from build123d import *

# Parameters (mm, degrees)
BOSS_EXTRUDE1_DEPTH = 77.15
CUT_EXTRUDE1_REACH  = 208.975
SKETCH2_R           = 1.75
SKETCH2_W           = 37
SKETCH2_H           = 18
FILLET1_R           = 2
FILLET2_R           = 10
SKETCH6_OUTSIDE_W   = 125.596
SKETCH6_OUTSIDE_H   = 125.596
SKETCH6_OUTSIDE_W_2 = 77.15
SKETCH6_OUTSIDE_H_2 = 77.15
SKETCH6_OUTSIDE_R   = 2.1
SKETCH6_OUTSIDE_R_2 = 2.55
CUT_EXTRUDE2_DEPTH  = 5


with BuildPart() as part:
    # Sketch1 → Boss-Extrude1 (new body)
    with BuildSketch(Plane.XY):
        Polygon((-29.117903226, 28.371290323), (-29.117903226, -48.778709677), (-24.117903226, -48.778709677), (-24.117903226, 23.371290323), (175.882096774, 23.371290323), (175.882096774, 28.371290323), align=None)
    extrude(amount=BOSS_EXTRUDE1_DEPTH)

    # Sketch2 → Cut-Extrude1 (cut, up to next)
    with BuildSketch(Plane(origin=(0, 28.371290323, 0), x_dir=(1, 0, 0), z_dir=(0, 1, 0)), mode=Mode.PRIVATE) as cut_extrude1_sk1:
        with Locations(Location((169.632096774, -38.575, 0), (0, 0, 180))):
            Circle(SKETCH2_R)
    cut_extrude1_tool1 = extrude(cut_extrude1_sk1.sketch, amount=-CUT_EXTRUDE1_REACH, mode=Mode.PRIVATE) & part.part
    # Sketch2 → Cut-Extrude1 (cut, up to next)
    with BuildSketch(Plane(origin=(0, 28.371290323, 0), x_dir=(1, 0, 0), z_dir=(0, 1, 0)), mode=Mode.PRIVATE) as cut_extrude1_sk2:
        with Locations(Location((117.632096774, -38.575, 0), (0, 0, 180))):
            Circle(SKETCH2_R)
    cut_extrude1_tool2 = extrude(cut_extrude1_sk2.sketch, amount=-CUT_EXTRUDE1_REACH, mode=Mode.PRIVATE) & part.part
    # Sketch2 → Cut-Extrude1 (cut, up to next)
    with BuildSketch(Plane(origin=(0, 28.371290323, 0), x_dir=(1, 0, 0), z_dir=(0, 1, 0)), mode=Mode.PRIVATE) as cut_extrude1_sk3:
        Polygon((175.882096774, -13.575), (115.882096774, -13.575), (-29.117903226, 0), (175.882096774, 0), align=None)
    cut_extrude1_tool3 = extrude(cut_extrude1_sk3.sketch, amount=-CUT_EXTRUDE1_REACH, mode=Mode.PRIVATE) & part.part
    # Sketch2 → Cut-Extrude1 (cut, up to next)
    with BuildSketch(Plane(origin=(0, 28.371290323, 0), x_dir=(1, 0, 0), z_dir=(0, 1, 0)), mode=Mode.PRIVATE) as cut_extrude1_sk4:
        Polygon((175.882096774, -63.575), (115.882096774, -63.575), (-29.117903226, -77.15), (175.882096774, -77.15), align=None)
    cut_extrude1_tool4 = extrude(cut_extrude1_sk4.sketch, amount=-CUT_EXTRUDE1_REACH, mode=Mode.PRIVATE) & part.part
    # Sketch2 → Cut-Extrude1 (cut, up to next)
    with BuildSketch(Plane(origin=(0, 28.371290323, 0), x_dir=(1, 0, 0), z_dir=(0, 1, 0)), mode=Mode.PRIVATE) as cut_extrude1_sk5:
        with Locations((146.882096774, -38.575)):
            Rectangle(SKETCH2_W, SKETCH2_H)
    cut_extrude1_tool5 = extrude(cut_extrude1_sk5.sketch, amount=-CUT_EXTRUDE1_REACH, mode=Mode.PRIVATE) & part.part
    add(cut_extrude1_tool1.solids().sort_by_distance((169.632097, 28.37129, 38.575))[0], mode=Mode.SUBTRACT)
    add(cut_extrude1_tool2.solids().sort_by_distance((117.632097, 28.37129, 38.575))[0], mode=Mode.SUBTRACT)
    add(cut_extrude1_tool3.solids().sort_by_distance((103.020462, 28.37129, 5.549528))[0], mode=Mode.SUBTRACT)
    add(cut_extrude1_tool4.solids().sort_by_distance((103.020462, 28.37129, 71.600472))[0], mode=Mode.SUBTRACT)
    add(cut_extrude1_tool5.solids().sort_by_distance((146.882097, 28.37129, 38.575))[0], mode=Mode.SUBTRACT)

    # Fillet1
    fillet1_edges = [part.edges().sort_by_distance(p)[0] for p in [
        (-29.117903226, 28.371290323, 38.575),
        (-24.117903226, 23.371290323, 38.575),
        (128.382096774, 25.871290323, 47.575),
        (128.382096774, 25.871290323, 29.575),
        (165.382096774, 25.871290323, 29.575),
        (165.382096774, 25.871290323, 47.575),
    ]]
    fillet(fillet1_edges, radius=FILLET1_R)

    # Fillet2
    fillet2_edges = [part.edges().sort_by_distance(p)[0] for p in [
        (175.882096774, 25.871290323, 13.575),
        (175.882096774, 25.871290323, 63.575),
    ]]
    fillet(fillet2_edges, radius=FILLET2_R)

    # Sketch6 outside → Cut-Extrude2 (cut)
    # profile 1 of 6: a face of its own
    with BuildSketch(Plane.ZY.offset(29.117903226)):
        with Locations((38.575, -10.204)):
            Rectangle(SKETCH6_OUTSIDE_W, SKETCH6_OUTSIDE_H)
        with Locations((38.575, -10.203709677)):
            Rectangle(SKETCH6_OUTSIDE_W_2, SKETCH6_OUTSIDE_H_2, mode=Mode.SUBTRACT)
    # profile 2 of 6: a face of its own
    with BuildSketch(Plane.ZY.offset(29.117903226)):
        with Locations((8.575, -20.203709677)):
            Circle(SKETCH6_OUTSIDE_R)
    # profile 3 of 6: a face of its own
    with BuildSketch(Plane.ZY.offset(29.117903226)):
        with Locations((8.575, -0.203709677)):
            Circle(SKETCH6_OUTSIDE_R)
    # profile 4 of 6: a face of its own
    with BuildSketch(Plane.ZY.offset(29.117903226)):
        with Locations((38.575, -40.203709677)):
            Circle(SKETCH6_OUTSIDE_R_2)
    # profile 5 of 6: a face of its own
    with BuildSketch(Plane.ZY.offset(29.117903226)):
        with Locations((68.575, -20.203709677)):
            Circle(SKETCH6_OUTSIDE_R)
    # profile 6 of 6: a face of its own
    with BuildSketch(Plane.ZY.offset(29.117903226)):
        with Locations((68.575, -0.203709677)):
            Circle(SKETCH6_OUTSIDE_R)
    extrude(amount=-CUT_EXTRUDE2_DEPTH, mode=Mode.SUBTRACT)


solid = part.part
Check sheet for the modelled part. Datum: model origin and axes. Units: mm. A direction names the side the tool comes from. Round coordinates to 2 decimals unless told otherwise and drop trailing zeros. Order: outer loops, then holes, each group sorted by start corner. A loop starts at its lowest first (then second) coordinate and runs counter-clockwise, first axis right, second up.
Q1. Draft check along Z on faces 5 (the face through (119.38, 25.91, 38.65)), 6 (the face through (167.963, 25.906, 39.101)), 7 (the face through (141, 26, 63.575)), 8 (the face through (-27, -48.779, 38)). Enter one of: pulls with the +Z half, pulls with the -Z half, needs draft (parallel to the pull), parting line crosses it, or undercut.
Filled sheet:
face 5: undercut
face 6: undercut
face 7: pulls with the +Z half
face 8: needs draft
Q2. Scan lines: L1, parallel to Z at x = 137.5, y = 24 (3 decimals); L2, parallel to Y at x = -9, z = 34; L3, parallel to X at y = -10.5, z = 7. Record each from-to range of solid material in increasing order.
Filled sheet:
L1: z = 13.575 to 29.575, 47.575 to 63.575
L2: y = 23.37 to 28.37
L3: x = -29.12 to -24.12
Q3. Cross-section at C-C, the plane y = 5.5. Enter the section's corners in (x, z), plus the area to 3 significant figures.
Filled sheet:
outline: (-29.12, 0) - (-24.12, 0.47) - (-24.12, 76.68) - (-29.12, 77.15) - close
area: 383 mm2
Q4. Set-up check for faces 1 (the face through (147, 26, 29.575)), 2 (the face through (141, 26, 13.575)), 3 (the face through (53, 28.371, 38)), 4 (the face through (-24.118, -14, 38)): record each of +Z, -Z, +X, -X, +Y, -Y from which the full face is reachable in a straight line by a thin tool's end or side.
Filled sheet:
face 1: +Y, -Y
face 2: -Z, +X, +Y, -Y
face 3: +Z, -Z, +X, -X, +Y
face 4: +Z, -Z, +X, -Y
Q5. Cross-section at A-A, the plane x = 142.5. Enter the section's corners in (y, z) (3 decimals).
Filled sheet:
outline: (23.371, 13.575) - (28.371, 13.575) - (28.371, 29.575) - (23.371, 29.575) - close; (23.371, 47.575) - (28.371, 47.575) - (28.371, 63.575) - (23.371, 63.575) - close
Q6. Cross-section at B-B, the plane z = 21. Enter the section's corners in (x, y).
Filled sheet:
outline: (-29.12, -48.78) - (-24.12, -48.78) - (-24.12, 21.37) arc R2 cw to (-22.12, 23.37) - (175.54, 23.37) - (175.54, 28.37) - (-27.12, 28.37) arc R2 ccw to (-29.12, 26.37) - close
Q7. Cross-section at D-D, the plane x = 63.5. Enter the section's corners in (y, z).
Filled sheet:
outline: (23.37, 8.67) - (28.37, 8.67) - (28.37, 68.48) - (23.37, 68.48) - close
Q8. Depth check by flat-ended pin: P1, Ø12, axis at y = 11, z = 57, coming from the +X side; P2, Ø4, axis at x = 169.63, z = 38.58, coming from the -Y side; P3, Ø4, axis at x = 117.63, z = 38.58, coming from the +Y side; P4, Ø1.5, axis at x = 149.5, y = 25.5, coming from the +Z side (3 decimals). Enter the tip coordinate at first touch or a pass-through.
Filled sheet:
P1: stops at x = -24.12
P2: stops at y = 23.37
P3: stops at y = 28.37
P4: stops at z = 63.575
